from build123d import *

# Parameters (mm, degrees)
BOSS_EXTRUDE1_DEPTH = 50.8
FILLET1_R           = 12.7
SHELL1_T            = -2.54
SKETCH2_R           = 8.636
CUT_EXTRUDE1_DEPTH  = 2.54


with BuildPart() as part:
    # Sketch1 → Boss-Extrude1 (new body)
    with BuildSketch(Plane(origin=(0, 0, 0), x_dir=(1, 0, 0), z_dir=(0, 1, 0))):
        with BuildLine():
            Line((-50.891439248, 0), (50.891439248, 0))
            ThreePointArc((50.891439248, 0), (56.033447259, 1.087517336), (60.29482175, 4.163818329))
            Line((60.29482175, 4.163818329), (140.996266194, 93.063818329))
            ThreePointArc((140.996266194, 93.063818329), (143.205366356, 106.742008011), (131.592883692, 114.3))
            Line((131.592883692, 114.3), (-131.592883692, 114.3))
            ThreePointArc((-131.592883692, 114.3), (-143.205366356, 106.742008011), (-140.996266194, 93.063818329))
            Line((-140.996266194, 93.063818329), (-60.29482175, 4.163818329))
            ThreePointArc((-60.29482175, 4.163818329), (-56.033447259, 1.087517336), (-50.891439248, 0))
        make_face()
    extrude(amount=BOSS_EXTRUDE1_DEPTH)

    # Fillet1
    fillet1_edges = [part.edges().sort_by_distance(p)[0] for p in [
        (-56.033447259, 0, -1.087517336),
        (0, 0, 0),
        (56.033447259, 0, -1.087517336),
        (100.645543972, 0, -48.613818329),
        (143.205366356, 0, -106.742008011),
        (0, 0, -114.3),
        (-143.205366356, 0, -106.742008011),
        (-100.645543972, 0, -48.613818329),
    ]]
    fillet(fillet1_edges, radius=FILLET1_R)

    # Shell1
    shell1_openings = [part.faces().sort_by_distance(p)[0] for p in [
        (0, 50.8, -65.668899596),
    ]]
    offset(amount=SHELL1_T, openings=shell1_openings, kind=Kind.INTERSECTION)

    # Sketch2 → Cut-Extrude1 (cut)
    with BuildSketch(Plane.XZ):
        with Locations(Location((-26.127205075, -88.9, 0), (0, 0, 270))):
            Circle(SKETCH2_R)
    extrude(amount=-CUT_EXTRUDE1_DEPTH, mode=Mode.SUBTRACT)


solid = part.part
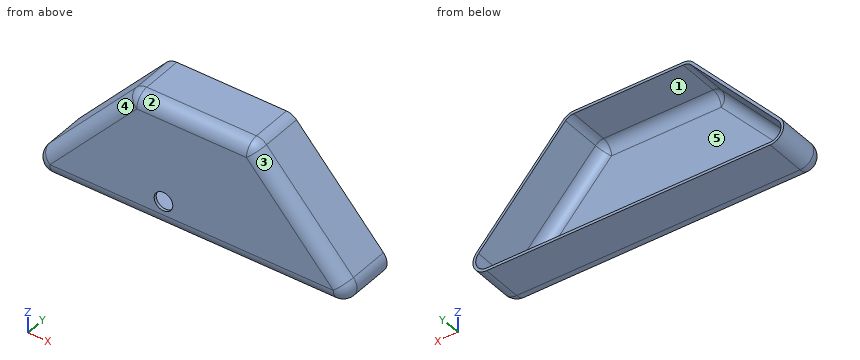
CAD build for the part. Positions are in the model's coordinates, mm. Face numbers are marked on the shaded views. A direction names the side the tool comes from. Coordinates: 2 decimals unless noted, no trailing zeros. Loops run counter-clockwise (first coordinate to the right, second up) from the corner with the lowest first, then second, coordinate; pieces in that order, holes last. Notation, with made-up numbers: (50, 61.5) -> (87, 61.5) arc R13 ccw to (87, 67.5) -> close; hole circle Ø6 at (72, 11.25). An arc over 180 degrees is marked (long way). One line per item, written item: value.
1. Drill centre lines: line 1 (X direction, y = 45, z = -102) (3 decimals); line 2 (Z direction, x = -52, y = 40); line 3 (Z direction, x = 2, y = 49). Where is each one in solid material? Low to high. Write a range as [from, to].
Answers:
line 1: x = [-144.287, -141.745], [141.745, 144.287]
line 2: z = [-114.3, -111.76], [-2.6, -0.05]
line 3: z = [-114.3, -111.76], [-2.54, 0]
2. Slice it at C-C on y = 9. Write the cut outline in (x, z), and give its area (3 significant figures).
Answers:
outline: (-140.59, -93.43) arc R12.15 ccw to (-131.59, -113.75) -> (131.59, -113.75) arc R12.15 ccw to (140.59, -93.43) -> (59.89, -4.53) arc R12.15 ccw to (50.89, -0.55) -> (-50.89, -0.55) arc R12.15 ccw to (-59.89, -4.53) -> close; hole (-138.6, -95.24) arc R9.46 ccw to (-131.59, -111.06) -> (131.59, -111.06) arc R9.46 ccw to (138.6, -95.24) -> (57.9, -6.34) arc R9.46 ccw to (50.89, -3.24) -> (-50.89, -3.24) arc R9.46 ccw to (-57.9, -6.34) -> close
area: 1,810 mm^2
3. Flat gauge pins, fed straight in: P1, Ø2, axis at x = -99, y = 25, coming from the +Z side; P2, Ø12, axis at y = 29.5, z = -15.5, coming from the -X side; P3, Ø2, axis at x = -44.5, z = -35, coming from the +Y side; P4, Ø10.5, axis at x = -26.13, z = -88.9, coming from the +Y side. Where does each tip first touch, or does it go through?
Answers:
P1: stops at z = -45.7
P2: stops at x = -76.03
P3: stops at y = 2.54
P4: passes through
4. Slice it at A-A on y = 27. Write the cut outline in (x, z), and give its area (3 significant figures).
Answers:
outline: (-141, -93.06) arc R12.7 ccw to (-131.59, -114.3) -> (131.59, -114.3) arc R12.7 ccw to (141, -93.06) -> (60.29, -4.16) arc R12.7 ccw to (50.89, 0) -> (-50.89, 0) arc R12.7 ccw to (-60.29, -4.16) -> close; hole (-139.12, -94.77) arc R10.16 ccw to (-131.59, -111.76) -> (131.59, -111.76) arc R10.16 ccw to (139.12, -94.77) -> (58.41, -5.87) arc R10.16 ccw to (50.89, -2.54) -> (-50.89, -2.54) arc R10.16 ccw to (-58.41, -5.87) -> close
area: 1,720 mm^2
5. Pull direction X, two halves, no side cores. Call the marked faces 1, 2 and 3: pulls with the +X half, pulls with the -X half, needs draft (parallel to the pull), parting line crosses it, or undercut.
Answers:
face 1: undercut
face 2: needs draft
face 3: pulls with the +X half
6. Which spindle directions (+Z, -Z, +X, -X, +Y, -Y) get a long thin tool onto all of the face, cutting with end or side? Do the marked faces 4 and 5. Say none if no direction does.
Answers:
face 4: +Z, -X, -Y
face 5: +Y
7. Slice it at B-B on x = 38. Write the cut outline in (y, z).
Answers:
outline: (0, -101.6) arc R12.7 ccw to (12.7, -114.3) -> (50.8, -114.3) -> (50.8, -111.76) -> (12.7, -111.76) arc R10.16 cw to (2.54, -101.6) -> (2.54, -12.7) arc R10.16 cw to (12.7, -2.54) -> (50.8, -2.54) -> (50.8, 0) -> (12.7, 0) arc R12.7 ccw to (0, -12.7) -> close
